Part model, mm, in its own coordinate system. A direction names the side the tool comes from. Round coordinates to 2 decimals unless told otherwise and drop trailing zeros. Loops run counter-clockwise (first coordinate to the right, second up) from the corner with the lowest first, then second, coordinate; pieces in that order, holes last. Notation, with made-up numbers: M -26,43 L 24,43 A22 ccw 24,50 Z; hole C -18,27 d5. An arc over 180 degrees is marked long. Put each result on its own line as item: value. Start each with the question number.
1) Slice it at D-D on y = 1. Give the cut face in (x, z).
2) Probe line 1 along X through (y, z) = (-2.5, 0); line 2 along X through (y, z) = (-0.8, 0); line 3 along Y through (x, z) = (18.5, -6.5). List the from-to ranges inside material, lowest first.
3) Slice it at C-C on y = -1.75. Give the cut face in (x, z).
4) Slice it at A-A on z = 0. Give the cut face in (x, y), then the cut area to 3 significant figures.
5) Which spindle directions (+Z, -Z, +X, -X, +Y, -Y) get a long thin tool onto all of the face, cutting with end or side? Do faces 4 (the cylindrical face through (21.35, -1.45, 14.14)), 5 (the flat face through (-22, 1, 2.5)), 6 (the flat face through (0, 1, -13.75)). Say none if no direction does.
6) Pull direction Z, two halves, no side cores. Call faces 1 (the flat face through (0, -2, -15)), 2 (the flat face through (-22.25, -2, 0)), 3 (the flat face through (4, 0, -6)): +Z half, -Z half, draft (parallel to the pull), parting line (faces both ways), or undercut.
7) Slice it at B-B on x = 0. Give the cut face in (y, z).
8) Drop flat-ended pins along their axis: pin 1 Ø7.5 at (x, z) = (0, 0) entering from -Y; pin 2 Ø14 at (x, z) = (10, 5) entering from +Y; pin 3 Ø2 at (y, z) = (1.5, 0.5) entering from -X; pin 4 Ø0.7 at (x, z) = (-21.5, 0) entering from +Y. Give the stop position or say it passes through.
```python
from build123d import *

# Parameters (mm, degrees)
SKETCH1_W           = 44.5
SKETCH1_H           = 30
BOSS_EXTRUDE1_DEPTH = 5
CUT_EXTRUDE1_REACH  = 7
SKETCH2_R           = 4.5
SKETCH5_W           = 44.5
SKETCH5_H           = 30
SKETCH5_W_2         = 41.7
SKETCH5_H_2         = 27.5
BOSS_EXTRUDE2_DEPTH = 2
CUT_EXTRUDE5_REACH  = 46.5
SKETCH6_W           = 5
SKETCH6_H           = 1.6
FILLET1_R           = 3
SKETCH7_R           = 6.25
CUT_EXTRUDE6_DEPTH  = 1


with BuildPart() as part:
    # Sketch1 → Boss-Extrude1 (new body)
    with BuildSketch(Plane(origin=(0, 0, 0), x_dir=(1, 0, 0), z_dir=(0, 1, 0))):
        Rectangle(SKETCH1_W, SKETCH1_H)
    extrude(amount=-BOSS_EXTRUDE1_DEPTH)

    # Sketch2 → Cut-Extrude1 (cut, up to next)
    with BuildSketch(Plane(origin=(0, 0, 0), x_dir=(1, 0, 0), z_dir=(0, 1, 0)), mode=Mode.PRIVATE) as cut_extrude1_sk1:
        Circle(SKETCH2_R)
    cut_extrude1_tool1 = extrude(cut_extrude1_sk1.sketch, amount=-CUT_EXTRUDE1_REACH, mode=Mode.PRIVATE) & part.part
    add(cut_extrude1_tool1.solids().sort_by_distance((0, 0, 0))[0], mode=Mode.SUBTRACT)

    # Sketch5 → Boss-Extrude2 (add)
    with BuildSketch(Plane(origin=(0, 0, 0), x_dir=(1, 0, 0), z_dir=(0, 1, 0))):
        Rectangle(SKETCH5_W, SKETCH5_H)
        Rectangle(SKETCH5_W_2, SKETCH5_H_2, mode=Mode.SUBTRACT)
    extrude(amount=BOSS_EXTRUDE2_DEPTH)

    # Sketch6 → Cut-Extrude5 (cut, up to next)
    with BuildSketch(Plane.ZY.offset(22.25), mode=Mode.PRIVATE) as cut_extrude5_sk1:
        with Locations((0, 1.2)):
            Rectangle(SKETCH6_W, SKETCH6_H)
    cut_extrude5_tool1 = extrude(cut_extrude5_sk1.sketch, amount=-CUT_EXTRUDE5_REACH, mode=Mode.PRIVATE) & part.part
    add(cut_extrude5_tool1.solids().sort_by_distance((-22.25, 1.2, 0))[0], mode=Mode.SUBTRACT)

    # Fillet1
    fillet1_edges = [part.edges().sort_by_distance(p)[0] for p in [
        (-20.85, 1, 13.75),
        (20.85, 1, 13.75),
        (20.85, 1, -13.75),
        (-20.85, 1, -13.75),
        (22.25, -1.5, 15),
        (-22.25, -1.5, 15),
        (-22.25, -1.5, -15),
        (22.25, -1.5, -15),
    ]]
    fillet(fillet1_edges, radius=FILLET1_R)

    # Sketch7 → Cut-Extrude6 (cut)
    with BuildSketch(Plane(origin=(0, 0, 0), x_dir=(1, 0, 0), z_dir=(0, 1, 0))):
        Circle(SKETCH7_R)
    extrude(amount=-CUT_EXTRUDE6_DEPTH, mode=Mode.SUBTRACT)


solid = part.part
```
Recorded:
1. outline: M -22.25,-12 A3 ccw -19.25,-15 L 19.25,-15 A3 ccw 22.25,-12 L 22.25,12 A3 ccw 19.25,15 L -19.25,15 A3 ccw -22.25,12 L -22.25,2.5 L -20.85,2.5 L -20.85,10.75 A3 cw -17.85,13.75 L 17.85,13.75 A3 cw 20.85,10.75 L 20.85,-10.75 A3 cw 17.85,-13.75 L -17.85,-13.75 A3 cw -20.85,-10.75 L -20.85,-2.5 L -22.25,-2.5 Z
2. line 1: x = -22.25 to -4.5, 4.5 to 22.25
2. line 2: x = -22.25 to -6.25, 6.25 to 22.25
2. line 3: y = -5 to 0
3. outline: M -22.25,-12 A3 ccw -19.25,-15 L 19.25,-15 A3 ccw 22.25,-12 L 22.25,12 A3 ccw 19.25,15 L -19.25,15 A3 ccw -22.25,12 Z; hole C 0,0 d9
4. outline: M -22.25,-5 L -4.5,-5 L -4.5,-1 L -6.25,-1 L -6.25,0 L -20.85,0 L -20.85,0.4 L -22.25,0.4 Z; M 4.5,-5 L 22.25,-5 L 22.25,2 L 20.85,2 L 20.85,0 L 6.25,0 L 6.25,-1 L 4.5,-1 Z
4. area: 177 mm2
5. face 4: +Z, +X, +Y, -Y
5. face 5: -X, +Y
5. face 6: +Y
6. face 1: -Z half
6. face 2: draft
6. face 3: undercut
7. outline: M -5,-15 L 2,-15 L 2,-13.75 L 0,-13.75 L 0,-6.25 L -1,-6.25 L -1,-4.5 L -5,-4.5 Z; M -5,4.5 L -1,4.5 L -1,6.25 L 0,6.25 L 0,13.75 L 2,13.75 L 2,15 L -5,15 Z
8. pin 1: passes through
8. pin 2: stops at y = 0
8. pin 3: stops at x = 20.85
8. pin 4: stops at y = 0.4
